```python
from build123d import *

# Parameters (mm, degrees)
ESQUISSE1_R      = 9
ESQUISSE1_R_2    = 15
ESQUISSE1_R_3    = 1.5
EXTRUSION1_DEPTH = 3
ESQUISSE2_R      = 9
EXTRUSION2_DEPTH = 38.5
ESQUISSE3_R      = 15
EXTRUSION3_DEPTH = 34.5


with BuildPart() as part:
    # Esquisse1 → Extrusion1 (new body)
    with BuildSketch(Plane.XY):
        with BuildLine():
            Line((0, 0), (0, 55))
            ThreePointArc((0, 55), (20, 75), (40, 55))
            Line((40, 55), (40, 0))
            ThreePointArc((40, 0), (20, -20), (0, 0))
        make_face()
        with Locations((20, 55)):
            Circle(ESQUISSE1_R, mode=Mode.SUBTRACT)
        with Locations((20, 0)):
            Circle(ESQUISSE1_R_2, mode=Mode.SUBTRACT)
        with Locations((20, 68)):
            Circle(ESQUISSE1_R_3, mode=Mode.SUBTRACT)
        with Locations((20, 42)):
            Circle(ESQUISSE1_R_3, mode=Mode.SUBTRACT)
        with Locations((7, 55)):
            Circle(ESQUISSE1_R_3, mode=Mode.SUBTRACT)
        with Locations((33, 55)):
            Circle(ESQUISSE1_R_3, mode=Mode.SUBTRACT)
    extrude(amount=EXTRUSION1_DEPTH)

    # Esquisse2 → Extrusion2 (add)
    with BuildSketch(Plane.XY.offset(3)):
        with BuildLine():
            Line((0, 0), (0, 23.278556149))
            ThreePointArc((0, 23.278556149), (13.490708127, 18.069265925), (27.949470784, 18.352272727))
            ThreePointArc((27.949470784, 18.352272727), (30.977490249, -16.718095222), (0, 0))
        make_face()
        with Locations((20, 0)):
            Circle(ESQUISSE2_R, mode=Mode.SUBTRACT)
    extrude(amount=-EXTRUSION2_DEPTH)

    # Esquisse3 → Extrusion3 (cut)
    with BuildSketch(Plane.XY.offset(3)):
        with Locations((20, 0)):
            Circle(ESQUISSE3_R)
    extrude(amount=-EXTRUSION3_DEPTH, mode=Mode.SUBTRACT)


solid = part.part
```
CAD build for the part. Positions are in the model's coordinates, mm. A direction names the side the tool comes from. Give positions to 0.01 mm unless a question says otherwise; leave off trailing zeros. Order: outer loops, then holes, each group sorted by start corner. A loop starts at its lowest first (then second) coordinate and runs counter-clockwise, first axis right, second up.
(1) Saw through at B-B, the plane x = 24.5. Give the cut face in (y, z).
(2) Tool access for faces 1 (the flat face through (20, 28, 3)), 2 (the cylindrical face through (31.476, -16.38, -15.98)), 3 (the cylindrical face through (13.29, 18.105, -17.502)), 4 (the flat face through (26.5, -6.5, -31.5)): list every direction of +Z, -Z, +X, -X, +Y, -Y with a clear straight run to the whole face (end or side of a thin tool).
(3) Flat gauge pins, fed straight in: pin 1 (6 mm diameter, centred on x = 12, y = -8, fed in from +Z); pin 2 (4 mm diameter, centred on x = 20, y = 68, fed in from +Z); pin 3 (2.5 mm diameter, centred on x = 33, y = 55, fed in from +Z) (1 decimal); pin 4 (1 mm diameter, centred on x = 30.5, z = -28, fed in from +Y). Where does each tip first touch, or does it go through?
(4) Saw through at D-D, the plane x = 33. Give the cut face in (y, z).
(5) Mould opens along X. For faces 5 (the flat face through (11, -3, -35.5)), 6 (the flat face through (40, 28, 1)), 7 (the cylindrical face through (20, 75, 1)), 8 (the cylindrical face through (31.5, 55.07, 1.48)) say: released by +X, released by -X, zero draft, split by the parting line, or undercut.
(6) Drill centre lines: L1, parallel to Y at x = 20, z = 1; L2, parallel to Y at x = 33, z = 1; L3, parallel to Z at x = 19.5, y = 31. Where is each one in solid material? Low to high.
(7) Saw through at C-C, the plane x = 20. Give the cut face in (y, z), then the cut area to 3 significant figures.
(8) Saw through at A-A, the plane y = 42. Give the cut face in (x, z).
Results found:
1. outline: (-19.49, -35.5) - (-7.79, -35.5) - (-7.79, -31.5) - (-14.31, -31.5) - (-14.31, 3) - (-19.49, 3) - close; (7.79, -35.5) - (17.77, -35.5) - (17.77, 0) - (47.21, 0) - (47.21, 3) - (14.31, 3) - (14.31, -31.5) - (7.79, -31.5) - close; (62.79, 0) - (74.49, 0) - (74.49, 3) - (62.79, 3) - close
2. face 1: +Z, +X, -X, +Y, -Y
2. face 2: -Z
2. face 3: -Z, +Y
2. face 4: +Z
3. pin 1: stops at z = -31.5
3. pin 2: stops at z = 3
3. pin 3: passes through
3. pin 4: stops at y = 17.32
4. outline: (-15.2, -35.5) - (15.2, -35.5) - (15.2, 0) - (53.5, 0) - (53.5, 3) - (7.48, 3) - (7.48, -31.5) - (-7.48, -31.5) - (-7.48, 3) - (-15.2, 3) - close; (56.5, 0) - (70.2, 0) - (70.2, 3) - (56.5, 3) - close
5. face 5: zero draft
5. face 6: released by +X
5. face 7: split by the parting line
5. face 8: undercut
6. L1: y = -20 to -15, 15 to 40.5, 43.5 to 46, 64 to 66.5, 69.5 to 75
6. L2: y = -15.2 to -7.48, 7.48 to 53.5, 56.5 to 70.2
6. L3: z = 0 to 3
7. outline: (-20, -35.5) - (-9, -35.5) - (-9, -31.5) - (-15, -31.5) - (-15, 3) - (-20, 3) - close; (9, -35.5) - (17.5, -35.5) - (17.5, 0) - (40.5, 0) - (40.5, 3) - (15, 3) - (15, -31.5) - (9, -31.5) - close; (43.5, 0) - (46, 0) - (46, 3) - (43.5, 3) - close; (64, 0) - (66.5, 0) - (66.5, 3) - (64, 3) - close; (69.5, 0) - (75, 0) - (75, 3) - (69.5, 3) - close
7. area: 437 mm2
8. outline: (0, 0) - (18.5, 0) - (18.5, 3) - (0, 3) - close; (21.5, 0) - (40, 0) - (40, 3) - (21.5, 3) - close
